For this review, take the finished solid that the model builds, in its own axes (mm). A direction names the side the tool comes from. Coordinates: 2 decimals unless noted, no trailing zeros. Order: outer loops, then holes, each group sorted by start corner. A loop starts at its lowest first (then second) coordinate and runs counter-clockwise, first axis right, second up.
from build123d import *

# Parameters (mm, degrees)
SIDEPLATERIGHT_MIRRORED1_START       = -3
SIDEPLATERIGHT_MIRRORED1_OUTLINE_R   = 2.1
SIDEPLATERIGHT_MIRRORED1_OUTLINE_R_2 = 7
SIDEPLATERIGHT_MIRRORED1_DEPTH       = 3
BOSS_EXTRUDE1_DEPTH                  = 3
FILLET1_R                            = 40
SKETCH3_R                            = 2.1
CUT_EXTRUDE1_DEPTH                   = 3
CUT_EXTRUDE3_DEPTH                   = 274.658546368
CUT_EXTRUDE3_DEPTH_BACK              = 274.658546368
SKETCH5_W                            = 336
SKETCH5_H                            = 4


# Read off the part's stored shape, not the designer's step: sidePlateRight_Mirrored1
with BuildPart() as part:
    # sidePlateRight_Mirrored1 outline → sidePlateRight_Mirrored1 (new body)
    with BuildSketch(Plane(origin=(0, 0, 0), x_dir=(1, 0, 0), z_dir=(0, 1, 0)).offset(SIDEPLATERIGHT_MIRRORED1_START)):
        with BuildLine():
            Line((168, -39), (168, 206))
            ThreePointArc((168, 206), (165.071067812, 213.071067812), (158, 216))
            Line((158, 216), (-23, 216))
            Line((-23, 216), (-23, 60))
            ThreePointArc((-23, 60), (-24.171572875, 57.171572875), (-27, 56))
            Line((-27, 56), (-158, 56))
            ThreePointArc((-158, 56), (-165.071067812, 53.071067812), (-168, 46))
            Line((-168, 46), (-168, -39))
            Line((-168, -39), (168, -39))
        make_face()
        with BuildLine():
            ThreePointArc((-87.5, -27.189984024), (-88.671572875, -30.018411149), (-91.5, -31.189984024))
            Line((-91.5, -31.189984024), (-99.5, -31.189984024))
            ThreePointArc((-99.5, -31.189984024), (-102.328427125, -30.018411149), (-103.5, -27.189984024))
            Line((-103.5, -27.189984024), (-103.5, 24))
            ThreePointArc((-103.5, 24), (-104.671572875, 26.828427125), (-107.5, 28))
            Line((-107.5, 28), (-126.109686491, 28))
            ThreePointArc((-126.109686491, 28), (-128.938113615, 29.171572876), (-130.109686491, 32))
            Line((-130.109686491, 32), (-130.109686491, 40))
            ThreePointArc((-130.109686491, 40), (-128.938113615, 42.828427124), (-126.109686491, 44))
            Line((-126.109686491, 44), (-64.890313509, 44))
            ThreePointArc((-64.890313509, 44), (-62.061886384, 42.828427124), (-60.890313509, 40))
            Line((-60.890313509, 40), (-60.890313509, 32))
            ThreePointArc((-60.890313509, 32), (-62.061886384, 29.171572876), (-64.890313509, 28))
            Line((-64.890313509, 28), (-83.5, 28))
            ThreePointArc((-83.5, 28), (-86.328427125, 26.828427125), (-87.5, 24))
            Line((-87.5, 24), (-87.5, -27.189984024))
        make_face(mode=Mode.SUBTRACT)
        with Locations((-16, -8)):
            Circle(SIDEPLATERIGHT_MIRRORED1_OUTLINE_R, mode=Mode.SUBTRACT)
        with Locations((-16, 8)):
            Circle(SIDEPLATERIGHT_MIRRORED1_OUTLINE_R, mode=Mode.SUBTRACT)
        with Locations((16, -8)):
            Circle(SIDEPLATERIGHT_MIRRORED1_OUTLINE_R, mode=Mode.SUBTRACT)
        Circle(SIDEPLATERIGHT_MIRRORED1_OUTLINE_R_2, mode=Mode.SUBTRACT)
        with Locations((16, 8)):
            Circle(SIDEPLATERIGHT_MIRRORED1_OUTLINE_R, mode=Mode.SUBTRACT)
        with BuildLine():
            ThreePointArc((60, 36), (48, 48), (60, 60))
            Line((60, 60), (132, 60))
            ThreePointArc((132, 60), (144, 48), (132, 36))
            Line((132, 36), (60, 36))
        make_face(mode=Mode.SUBTRACT)
        with Locations((-16, 184)):
            Circle(SIDEPLATERIGHT_MIRRORED1_OUTLINE_R, mode=Mode.SUBTRACT)
        with Locations((-16, 200)):
            Circle(SIDEPLATERIGHT_MIRRORED1_OUTLINE_R, mode=Mode.SUBTRACT)
        with Locations((-16, 208)):
            Circle(SIDEPLATERIGHT_MIRRORED1_OUTLINE_R, mode=Mode.SUBTRACT)
        with BuildLine():
            ThreePointArc((60, 101), (48, 113), (60, 125))
            Line((60, 125), (132, 125))
            ThreePointArc((132, 125), (144, 113), (132, 101))
            Line((132, 101), (60, 101))
        make_face(mode=Mode.SUBTRACT)
        with Locations((16, 184)):
            Circle(SIDEPLATERIGHT_MIRRORED1_OUTLINE_R, mode=Mode.SUBTRACT)
        with Locations((16, 200)):
            Circle(SIDEPLATERIGHT_MIRRORED1_OUTLINE_R, mode=Mode.SUBTRACT)
        with Locations((16, 208)):
            Circle(SIDEPLATERIGHT_MIRRORED1_OUTLINE_R, mode=Mode.SUBTRACT)
        with BuildLine():
            ThreePointArc((60, 166), (48, 178), (60, 190))
            Line((60, 190), (132, 190))
            ThreePointArc((132, 190), (144, 178), (132, 166))
            Line((132, 166), (60, 166))
        make_face(mode=Mode.SUBTRACT)
    extrude(amount=SIDEPLATERIGHT_MIRRORED1_DEPTH)

    # Sketch1 → Boss-Extrude1 (add)
    with BuildSketch(Plane(origin=(0, 0, 0), x_dir=(1, 0, 0), z_dir=(0, 1, 0))):
        with BuildLine():
            Line((-168, 46), (-168, 151.833913223))
            ThreePointArc((-168, 151.833913223), (-161.957805488, 169.890035626), (-146.265096253, 180.672917782))
            Line((-146.265096253, 180.672917782), (-23, 216))
            Line((-23, 216), (-23, 46))
            Line((-23, 46), (-168, 46))
        make_face()
        with BuildLine():
            Line((-132, 93.668808042), (-60, 93.668808042))
            ThreePointArc((-60, 93.668808042), (-48, 81.668808042), (-60, 69.668808042))
            Line((-60, 69.668808042), (-132, 69.668808042))
            ThreePointArc((-132, 69.668808042), (-144, 81.668808042), (-132, 93.668808042))
        make_face(mode=Mode.SUBTRACT)
        with BuildLine():
            Line((-132, 158.668808042), (-60, 158.668808042))
            ThreePointArc((-60, 158.668808042), (-48, 146.668808042), (-60, 134.668808042))
            Line((-60, 134.668808042), (-132, 134.668808042))
            ThreePointArc((-132, 134.668808042), (-144, 146.668808042), (-132, 158.668808042))
        make_face(mode=Mode.SUBTRACT)
    extrude(amount=-BOSS_EXTRUDE1_DEPTH)

    # Fillet1
    fillet1_edges = [part.edges().sort_by_distance(p)[0] for p in [
        (-23, -1.5, -216),
    ]]
    fillet(fillet1_edges, radius=FILLET1_R)

    # Sketch3 → Cut-Extrude1 (cut)
    with BuildSketch(Plane(origin=(0, 0, 0), x_dir=(1, 0, 0), z_dir=(0, 1, 0))):
        with Locations(Location((-120, 17, 0), (0, 0, 270))):
            Circle(SKETCH3_R)
        with Locations(Location((-72, 17, 0), (0, 0, 270))):
            Circle(SKETCH3_R)
    extrude(amount=-CUT_EXTRUDE1_DEPTH, mode=Mode.SUBTRACT)

    # Sketch5 → Cut-Extrude3 (cut, two sides: drawn at the far end of the back side and taken through both)
    with BuildSketch(Plane(origin=(0, 0, 0), x_dir=(1, 0, 0), z_dir=(0, 1, 0)).offset(-CUT_EXTRUDE3_DEPTH_BACK)):
        with Locations((0, -37)):
            Rectangle(SKETCH5_W, SKETCH5_H)
    extrude(amount=CUT_EXTRUDE3_DEPTH + CUT_EXTRUDE3_DEPTH_BACK, mode=Mode.SUBTRACT)


solid = part.part
1. Take a section at A-A, the plane x = 0. Give the boundary of the cut face in (y, z), plus the area to 3 significant figures.
Answer below:
outline: (-3, -216) - (0, -216) - (0, -7) - (-3, -7) - close; (-3, 7) - (0, 7) - (0, 35) - (-3, 35) - close
area: 711 mm2
2. Clearance check with flat-ended pins moving along their axes: pin 1 Ø1.5 at (x, y) = (-77, -1) entering from -Z; pin 2 Ø1.5 at (x, y) = (-108.5, -2) entering from -Z; pin 3 Ø1.5 at (x, y) = (-118, -1) entering from -Z. State where each tip first meets the part, or that it passes through.
Answer below:
pin 1: stops at z = -200.74
pin 2: stops at z = -191.71
pin 3: stops at z = -188.99
3. To check wall thickness, follow L1, parallel to X at y = -1.85, z = 8; L2, parallel to Z at x = 16, y = -0.7; L3, parallel to X at y = -2.1, z = -1. State the ranges of each line that lie inside material, in increasing order.
Answer below:
L1: x = -168 to -103.5, -87.5 to -18.1, -13.9 to 13.9, 18.1 to 168
L2: z = -216 to -210.1, -205.9 to -202.1, -197.9 to -186.1, -181.9 to -10.1, -5.9 to 5.9, 10.1 to 35
L3: x = -168 to -103.5, -87.5 to -6.93, 6.93 to 168
4. Take a section at D-D, the plane x = -51.5. Give the boundary of the cut face in (y, z).
Answer below:
outline: (-3, -207.83) - (0, -207.83) - (0, -155.14) - (-3, -155.14) - close; (-3, -138.2) - (0, -138.2) - (0, -90.14) - (-3, -90.14) - close; (-3, -73.2) - (0, -73.2) - (0, 35) - (-3, 35) - close
5. Machinability: for faces 1 (the face through (48, -2, -48)), 2 (the face through (-88.158, -1.479, -197.326)), which of the approach directions +Z, -Z, +X, -X, +Y, -Y give a long, thin tool a straight path to every point of the face, cutting with its end or side? Answer none if there is none.
Answer below:
face 1: +Y, -Y
face 2: -Z, -X, +Y, -Y
6. The part is to be moulded in two halves that separate along X. For faces 3 (the face through (165.15, -1.52, -212.99)), 4 (the face through (144, -2, -178)), 5 (the face through (-162.1, -1.5, -169.7)), say which applies: +X half, -X half, draft (parallel to the pull), parting line (faces both ways), or undercut.
Answer below:
face 3: +X half
face 4: undercut
face 5: -X half
7. Take a section at C-C, the plane y = -0.7. Give the number of separate pieces and of enclosed holes in the cut face, plus the area to 3 significant figures.
Answer below:
separate pieces: 1
enclosed holes: 19
area: 67,900 mm2
8. Take a section at B-B, the plane z = -48. Give the boundary of the cut face in (x, y).
Answer below:
outline: (-168, -3) - (48, -3) - (48, 0) - (-168, 0) - close; (144, -3) - (168, -3) - (168, 0) - (144, 0) - close
